Can you work these out from the model? Positions are in its coordinate system, mm. Face numbers are marked on the shaded views. A direction names the side the tool comes from. Give positions to 0.01 mm unless a question says otherwise; leave off trailing zeros. Order: outer loops, then holes, each group sorted by start corner. A loop starts at its lowest first (then second) coordinate and runs counter-clockwise, first axis right, second up.
Item 1: I want a section at A-A, the plane y = 1. Write out the boundary of the cut face in (x, z), then the cut area to 3 significant figures.
Item 2: If we mould it in two halves opening along X, with no side actions, what happens to the marked faces 4, 5, 6 and 7? For each: +X half, -X half, draft (parallel to the pull), parting line (faces both ways), or undercut.
Item 3: If I drill on line 1 along X through (y, z) = (13.25, -25.5); line 2 along X through (y, z) = (10.5, -12); line 3 along Z through (x, y) = (3.5, 5.75), over which ranges is the centre line in solid material (lowest first)?
Item 4: I'm going to push flat-ended pins straight in: pin 1 Ø1.5 at (x, z) = (22, -20) entering from -Y; pin 2 Ø3 at (x, z) = (18.5, -17.5) entering from -Y. Where does each tip first touch, or does it pass through?
Item 5: Which directions (+Z, -Z, +X, -X, +Y, -Y) give clear straight access to the entire face, cutting with the end or side of a thin tool? Please do the marked faces 1, 2 and 3.
Item 6: I want a section at B-B, the plane z = -9.5. Write out the boundary of the cut face in (x, y).
Item 7: I want a section at C-C, the plane x = 43.5. Write out the boundary of the cut face in (y, z), then the cut area to 3 significant figures.
Item 8: I want a section at D-D, the plane y = 4.5. Count the separate pieces of the cut face and the enclosed holes in it, then the cut area to 3 significant figures.
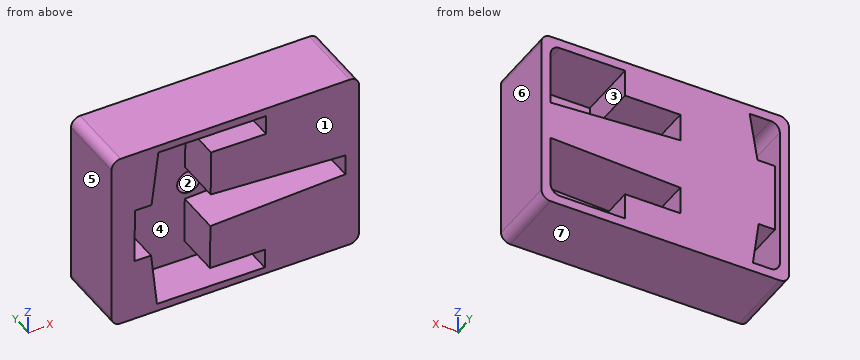
```python
from build123d import *

# Parameters (mm, degrees)
SKETCH1_W              = 54
SKETCH1_H              = 39.25
BOSS_EXTRUDE1_DEPTH    = 46.5
FILLET1_R              = 2
FILLET2_R              = 2
Z_95_START             = -0.023652431
Z_95_BLANK_DEPTH       = 10
Z_95_START_2           = -5.023652431
Z_95_BLANK_2_OUTLINE_R = 2.5
Z_95_BLANK_2_DEPTH     = 5
BODY_MOVE_COPY3_ANGLE  = 180
BODY_MOVE_COPY4_ANGLE  = 89.5
SKETCH4_W              = 54
SKETCH4_H              = 39.25
CUT_EXTRUDE1_DEPTH     = 31
CUT_EXTRUDE2_DEPTH     = 31
BOSS_EXTRUDE2_DEPTH    = 2
FILLET3_R              = 2
FILLET4_R              = 2
FILLET5_R              = 2
FILLET6_R              = 2


with BuildPart() as part:
    # Sketch1 → Boss-Extrude1 (new body)
    with BuildSketch(Plane(origin=(0, 0, 0), x_dir=(1, 0, 0), z_dir=(0, 1, 0))):
        with Locations((27, 19.625)):
            Rectangle(SKETCH1_W, SKETCH1_H)
    extrude(amount=BOSS_EXTRUDE1_DEPTH)

    # Fillet1
    fillet1_edges = [part.edges().sort_by_distance(p)[0] for p in [
        (0, 23.25, 0),
    ]]
    fillet(fillet1_edges, radius=FILLET1_R)

    # Fillet2
    fillet2_edges = [part.edges().sort_by_distance(p)[0] for p in [
        (0, 23.25, -39.25),
        (54, 23.25, -39.25),
        (54, 23.25, 0),
    ]]
    fillet(fillet2_edges, radius=FILLET2_R)


with BuildPart() as body_2:
    # Z-95 Blank: read off the stored shape, not the designer's step
    # Z-95 Blank outline → Z-95 Blank (new body)
    with BuildSketch(Plane(origin=(0, 0, 0), x_dir=(1, 0, 0), z_dir=(0, 1, 0)).offset(Z_95_START)):
        Polygon((-39.475833264, 51.689675598), (-39.475833264, 48.062948495), (-51.475833264, 46.678320586), (-51.475833264, 23.139646129), (-47.225833264, 23.139646129), (-47.225833264, 35.139646129), (-37.225833264, 35.139646129), (-35.725833264, 5.689675598), (-31.225833264, 5.689675598), (-29.725833264, 35.139646129), (-19.725833264, 35.139646129), (-19.725833264, 23.139646129), (-15.475833264, 23.139646129), (-15.475833264, 46.678320586), (-27.475833264, 48.062948495), (-27.475833264, 51.689675598), align=None)
    extrude(amount=Z_95_BLANK_DEPTH)

    # Z-95 Blank 2 outline → Z-95 Blank 2 (add)
    with BuildSketch(Plane(origin=(0, 0, 0), x_dir=(1, 0, 0), z_dir=(0, 1, 0)).offset(Z_95_START_2)):
        with Locations((-33.475833264, 34.343753809)):
            Circle(Z_95_BLANK_2_OUTLINE_R)
    extrude(amount=Z_95_BLANK_2_DEPTH)


with BuildPart() as body_2_1:
    # Body-Move/Copy3: moved
    add(body_2.part.rotate(Axis((0, 2.476347569, -28.689675598), (1, 0, 0)), BODY_MOVE_COPY3_ANGLE))


with BuildPart() as body_2_2:
    # Body-Move/Copy4: moved
    add(body_2_1.part.rotate(Axis((-33.475833264, 0, -28.689675598), (0, -1, 0)), BODY_MOVE_COPY4_ANGLE))


with BuildPart() as body_2_3:
    # Body-Move/Copy5: moved
    add(body_2_2.part.moved(Location((61.536777905, 5.06338101, 8.948981511))))


with BuildPart() as body_2_4:
    # Body-Move/Copy6: moved
    add(body_2_3.part.moved(Location((0, -0.229742035, 0))))


with BuildPart() as part_1:
    add(part.part)

    # Intersect1: read off the stored shape, not the designer's step
    # Intersect1: cut body 2
    add(body_2_4.part, mode=Mode.SUBTRACT)

    # Sketch4 → Cut-Extrude1 (cut)
    with BuildSketch(Plane(origin=(0, 46.5, 0), x_dir=(1, 0, 0), z_dir=(0, 1, 0))):
        with Locations((27, 19.625)):
            Rectangle(SKETCH4_W, SKETCH4_H)
    extrude(amount=-CUT_EXTRUDE1_DEPTH, mode=Mode.SUBTRACT)

    # Sketch5 → Cut-Extrude2 (cut)
    with BuildSketch(Plane(origin=(0, 0, 0), x_dir=(-1, 0, 0), z_dir=(0, -1, 0))):
        Polygon((-23.713680343, 7.952308665), (-23.713680343, 14.054528407), (-52, 15.742860627), (-52, 2), (-35.766082295, 2), (-35.766082295, 7.952308665), align=None)
        Polygon((-23.713680343, 25.345964802), (-23.713680343, 31.453203507), (-35.766082295, 31.453203507), (-35.766082295, 37.25), (-52, 37.25), (-52, 24.152615413), align=None)
        Polygon((-6.871546498, 12.395456139), (-8.594812047, 2), (-2, 2), (-2, 37.25), (-7.869100925, 37.25), (-6.622123507, 27.553904956), (-3.057950712, 27.553904956), (-3.057950712, 12.395456139), align=None)
    extrude(amount=-CUT_EXTRUDE2_DEPTH, mode=Mode.SUBTRACT)

    # Sketch6 → Boss-Extrude2 (add)
    with BuildSketch(Plane.XZ):
        Polygon((52, -24.152615413), (23.713680343, -25.345964802), (23.713680343, -31.453203507), (35.766082295, -31.453203507), (35.766082295, -37.25), (52, -37.25), align=None)
        Polygon((52, -15.742860627), (23.713680343, -14.054528407), (23.713680343, -7.952308665), (35.766082295, -7.952308665), (35.766082295, -2), (52, -2), align=None)
        Polygon((8.594812047, -2), (6.871546498, -12.395456139), (3.057950712, -12.395456139), (3.057950712, -27.553904956), (6.622123507, -27.553904956), (7.869100925, -37.25), (2, -37.25), (2, -2), align=None)
    extrude(amount=-BOSS_EXTRUDE2_DEPTH)

    # Fillet3
    fillet3_edges = [part_1.edges().sort_by_distance(p)[0] for p in [
        (52, 8.75, -2),
    ]]
    fillet(fillet3_edges, radius=FILLET3_R)

    # Fillet4
    fillet4_edges = [part_1.edges().sort_by_distance(p)[0] for p in [
        (2, 8.75, -2),
    ]]
    fillet(fillet4_edges, radius=FILLET4_R)

    # Fillet5
    fillet5_edges = [part_1.edges().sort_by_distance(p)[0] for p in [
        (52, 8.75, -37.25),
    ]]
    fillet(fillet5_edges, radius=FILLET5_R)

    # Fillet6
    fillet6_edges = [part_1.edges().sort_by_distance(p)[0] for p in [
        (2, 8.75, -37.25),
    ]]
    fillet(fillet6_edges, radius=FILLET6_R)


solid = part_1.part
```
Results list:
1. outline: (0, -37.25) arc R2 ccw to (2, -39.25) - (52, -39.25) arc R2 ccw to (54, -37.25) - (54, -2) arc R2 ccw to (52, 0) - (2, 0) arc R2 ccw to (0, -2) - close; hole (5.01, -25.54) - (8.64, -25.57) - (9.92, -37.58) - (33.45, -37.79) - (33.49, -33.54) - (21.49, -33.43) - (21.58, -23.43) - (51.04, -22.19) - (51.08, -17.69) - (21.64, -15.93) - (21.73, -5.93) - (33.73, -6.04) - (33.77, -1.79) - (10.23, -1.58) - (8.74, -13.57) - (5.11, -13.54) - close
1. area: 1,350 mm2
2. face 4: undercut
2. face 5: -X half
2. face 6: +X half
2. face 7: draft
3. line 1: x = 0 to 2, 3.06 to 23.71, 52 to 54
3. line 2: x = 0 to 2, 6.94 to 23.71, 52 to 54
3. line 3: z = -39.25 to -37.19, -27.55 to -12.4, -2.06 to 0
4. pin 1: stops at y = 14.81
4. pin 2: stops at y = 9.81
5. face 1: +Z, -Z, +X, -X, -Y
5. face 2: -Y
5. face 3: +Y
6. outline: (0, 0) - (9.25, 0) - (9.25, 9.81) - (21.7, 9.81) - (21.7, 0) - (54, 0) - (54, 15.5) - (52, 15.5) - (52, 2) - (23.71, 2) - (23.71, 15.5) - (7.35, 15.5) - (7.35, 2) - (2, 2) - (2, 15.5) - (0, 15.5) - close
7. outline: (0, -39.25) - (15.5, -39.25) - (15.5, -37.25) - (2, -37.25) - (2, -24.51) - (15.5, -24.51) - (15.5, -15.24) - (2, -15.24) - (2, -2) - (15.5, -2) - (15.5, 0) - (0, 0) - (0, -17.24) - (9.81, -17.24) - (9.81, -22.51) - (0, -22.51) - close
7. area: 206 mm2
8. separate pieces: 1
8. enclosed holes: 4
8. area: 645 mm2
